Autodesk Inventor part; units mm, degrees
ref_plane "YZ Plane" through (0, 0, 0) normal (1, 0, 0) x (0, 1, 0)
ref_plane "XZ Plane" through (0, 0, 0) normal (0, 1, 0) x (-1, 0, 0)
ref_plane "XY Plane" through (0, 0, 0) normal (0, 0, 1) x (1, 0, 0)
sketch "Sketch1" plane through (0, 0, 0) normal (0, 0, 1) x (1, 0, 0)
  arc A0 (72.4335, -68.9449) -> (-72.4335, -68.9449) centre (0, 0) ccw
  line L0 (0, 0) -> (0, -68.9449)
  arc A1 (75.8476, -68.9449) -> (-75.8476, -68.9449) centre (0, 0) ccw
  line L1 (0, 0) -> (88.7676, -51.25)
  line L2 (0, 0) -> (102.5, 0) construction
  line L3 (0, 0) -> (-88.7676, -51.25)
  line L4 (0, 0) -> (102.5, 0) construction
  line L5 (0, 0) -> (72.4784, 72.4784)
  line L6 (0, 0) -> (102.5, 0) construction
  line L7 (0, 0) -> (-72.4784, 72.4784)
  line L8 (0, 0) -> (102.5, 0) construction
  line L9 (0, 0) -> (-68.416, -39.5)
  line L10 (0, 0) -> (68.416, -39.5)
  line L11 (0, 0) -> (55.8614, 55.8614)
  line L12 (0, 0) -> (-55.8614, 55.8614)
  line L13 (-68.416, -39.5) -> (-51.416, -68.9449)
  line L14 (-68.416, -39.5) -> (-85.416, -10.0551)
  line L15 (68.416, -39.5) -> (51.416, -68.9449)
  line L16 (51.416, -68.9449) -> (68.416, -39.5)
  line L17 (68.416, -39.5) -> (85.416, -10.0551)
  line L18 (-51.416, -68.9449) -> (-75.8476, -68.9449)
  line L19 (-51.416, -68.9449) -> (51.416, -68.9449)
  line L20 (51.416, -68.9449) -> (75.8476, -68.9449)
  line L21 (85.416, -10.0551) -> (100.7418, -18.9035)
  line L22 (-85.416, -10.0551) -> (-100.7418, -18.9035)
  line L23 (-55.8614, 55.8614) -> (-79.9031, 31.8198)
  line L24 (-55.8614, 55.8614) -> (-31.8198, 79.9031)
  line L25 (55.8614, 55.8614) -> (79.9031, 31.8198)
  line L26 (55.8614, 55.8614) -> (31.8198, 79.9031)
  line L27 (-31.8198, 79.9031) -> (-44.3333, 92.4165)
  line L28 (-79.9031, 31.8198) -> (-92.4165, 44.3333)
  line L29 (31.8198, 79.9031) -> (44.3333, 92.4165)
  line L30 (79.9031, 31.8198) -> (92.4165, 44.3333)
  circle A2 centre (0, 0) radius 125
  line L31 (100.7418, -18.9035) -> (121.1717, -30.6987)
  line L32 (-100.7418, -18.9035) -> (-121.1717, -30.6987)
  line L33 (-92.4165, 44.3333) -> (-109.0975, 61.0142)
  line L34 (-44.3333, 92.4165) -> (-61.0142, 109.0975)
  line L35 (44.3333, 92.4165) -> (61.0142, 109.0975)
  line L36 (92.4165, 44.3333) -> (109.0975, 61.0142)
  circle A3 centre (0, 0) radius 120
  line L37 (-75.8476, -68.9449) -> (-104.267, -68.9449)
  line L38 (75.8476, -68.9449) -> (104.267, -68.9449)
  line L39 (68.416, -39.5) -> (86.416, -8.3231)
  line L40 (86.416, -8.3231) -> (121.6665, -28.675)
  line L41 (55.8614, 55.8614) -> (81.3173, 30.4056)
  line L42 (81.3173, 30.4056) -> (111.6152, 56.2764)
  line L43 (-68.416, -39.5) -> (-86.416, -8.3231)
  line L44 (-86.416, -8.3231) -> (-121.6665, -28.675)
  line L45 (-55.8614, 55.8614) -> (-81.3173, 30.4056)
  line L46 (-81.3173, 30.4056) -> (-110.0992, 59.1875)
  line L47 (-55.8614, 55.8614) -> (-30.4056, 81.3173)
  line L48 (-30.4056, 81.3173) -> (-59.1875, 110.0992)
  line L49 (55.8614, 55.8614) -> (30.4056, 81.3173)
  line L50 (30.4056, 81.3173) -> (59.1875, 110.0992)
  line L51 (68.416, -39.5) -> (50.416, -70.6769)
  line L52 (-68.416, -39.5) -> (-50.416, -70.6769)
  line L53 (51.416, -68.9449) -> (87.1717, -89.5884)
  line L54 (51.416, -68.9449) -> (92.7032, -68.9449) construction
  line L55 (50.416, -70.6769) -> (85.6665, -91.0288)
  line L56 (-50.416, -70.6769) -> (-85.6665, -91.0288)
  line L57 (-51.416, -68.9449) -> (-87.1717, -89.5884)
  point P0 (93.8835, 41.1356)
  point P1 (91.8949, 39.4376)
  point P2 (98.796, -15.4707)
  point P3 (101.1125, -16.8081)
  point P4 (40.5138, 91.4255)
  point P5 (42.4052, 93.3169)
  point P6 (-42.4052, 93.3169)
  point P7 (-40.5138, 91.4255)
  point P8 (-91.4255, 40.5138)
  point P9 (-93.3169, 42.4052)
  point P10 (-101.1125, -16.8081)
  point P11 (-98.796, -15.4707)
  point P12 (98.2171, -68.9449)
  point P13 (98.4432, -17.5764)
  point P14 (116.6644, -28.0964)
  point P15 (57.334, 105.4173)
  point P16 (105.4173, 57.334)
  point P17 (-105.4173, 57.334)
  point P18 (-57.334, 105.4173)
  point P19 (-98.2171, -68.9449)
  point P20 (-116.6644, -28.0964)
  point P21 (90.5398, 42.4565)
  point P22 (42.4565, 90.5398)
  point P23 (-42.4565, 90.5398)
  point P24 (-90.5398, 42.4565)
  point P25 (-98.4432, -17.5764)
  point P26 (-86.6025, -50)
  point P27 (-82.6644, -86.9862)
  point P28 (82.6644, -86.9862)
  dimension "d30" = 250
  dimension "d7" = 30
  dimension "d8" = 150
  dimension "d9" = 45
  dimension "d10" = 135
  dimension "d11" = 79
  dimension "d12" = 79
  dimension "d13" = 79
  dimension "d14" = 79
  dimension "d15" = 34
  dimension "d16" = 90
  dimension "d17" = 34
  dimension "d18" = 34
  dimension "d19" = 34
  dimension "d20" = 34
  dimension "d21" = 34
  dimension "d22" = 34
  dimension "d23" = 34
  dimension "d24" = 34
  dimension "d31" = 240
  dimension "d32" = 36
  dimension "d33" = 36
  dimension "d34" = 36
  dimension "d35" = 36
  dimension "d36" = 36
  dimension "d37" = 36
  dimension "d73" = 36
  dimension "d74" = 36
  dimension "d75" = 30
extrude "Extrusion3" add sketch "Sketch1" against normal blind 2 contours L20 L15 L1 A0 | A0 L1 A1 L20 | L1 L17 L21 A0 | A0 L21 A1 L1 | L19 L0 L1 L15 | L21 L39 L40 A0 | A0 L40 A1 L21 | L1 L5 L25 L41 L42 A0 L40 L39 L17 | L19 L13 L3 L0 | A0 L42 A1 L40 | L7 L24 L47 L48 A0 L50 L49 L26 L5 | L3 L14 L43 L44 A0 L46 L45 L23 L7 | L18 A0 L3 L13 | L42 L41 L30 A0 | A0 L30 A1 L42 | L3 A0 L22 L14 | L26 L29 A0 L5 | L5 A0 L30 L25 | L23 L28 A0 L7 | L7 A0 L27 L24 | L18 A1 L3 A0 | A0 L5 A1 L30 | L3 A1 L22 A0 | L22 A0 L44 L43 | A0 L29 A1 L5 | L49 L50 A0 L29 | L7 A1 L27 A0 | A0 L28 A1 L7 | L45 L46 A0 L28 | L27 A0 L48 L47 | L22 A1 L44 A0 | A0 L50 A1 L29 | L27 A1 L48 A0 | A0 L46 A1 L28 | L44 A1 L46 A0 | A0 L48 A1 L50
extrude "Extrusion4" add sketch "Sketch1" along normal blind 28 contours A0 L1 A1 L20 | A0 L21 A1 L1 | A0 L40 A1 L21 | A0 L42 A1 L40 | A0 L30 A1 L42 | L18 A1 L3 A0 | A0 L5 A1 L30 | L3 A1 L22 A0 | A0 L29 A1 L5 | L7 A1 L27 A0 | A0 L28 A1 L7 | L22 A1 L44 A0 | A0 L50 A1 L29 | L27 A1 L48 A0 | A0 L46 A1 L28 | L44 A1 L46 A0 | A0 L48 A1 L50
extrude "Extrusion5" add sketch "Sketch1" along normal blind 65 contours A0 L42 A1 L40 | L44 A1 L46 A0 | A0 L48 A1 L50
sketch "Sketch4" plane through (0, 0, -2) normal (0, 0, -1) x (-1, 0, 0)
  line L0 (0, 0) -> (-85, 0)
  line L1 (0, 0) -> (0, 85)
  line L2 (0, 0) -> (85, 0)
  circle A0 centre (-85, 0) radius 1.5
  circle A1 centre (0, 85) radius 1.5
  circle A2 centre (85, 0) radius 1.5
  circle A3 centre (0, 0) radius 75
  dimension "d60" = 85
  dimension "d61" = 85
  dimension "d62" = 85
  dimension "d63" = 3
  dimension "d64" = 3
  dimension "d65" = 3
  dimension "d66" = 150
extrude "Extrusion11" cut sketch "Sketch4" against normal blind 45
sketch "Sketch5" plane through (0, 0, -2) normal (0, 0, -1) x (-1, 0, 0)
  line L0 (72.4335, -68.9449) -> (-72.4335, -68.9449)
  line L1 (-72.4335, -68.9449) -> (-72.4335, -54.9449)
  line L2 (-72.4335, -54.9449) -> (129.3344, -54.9449)
  line L3 (129.3344, -54.9449) -> (-118.857, -54.9449)
  line L4 (-118.857, -54.9449) -> (-118.857, -84.9238)
  line L5 (-118.857, -84.9238) -> (129.3344, -84.9238)
  line L6 (129.3344, -84.9238) -> (129.3344, -54.9449)
  point P0 (0, 0)
  point P1 (-41.6566, -68.9449)
  dimension "d70" = 14
extrude "Extrusion12" cut sketch "Sketch5" against normal blind 4
properties part number "Falda-Parte1"
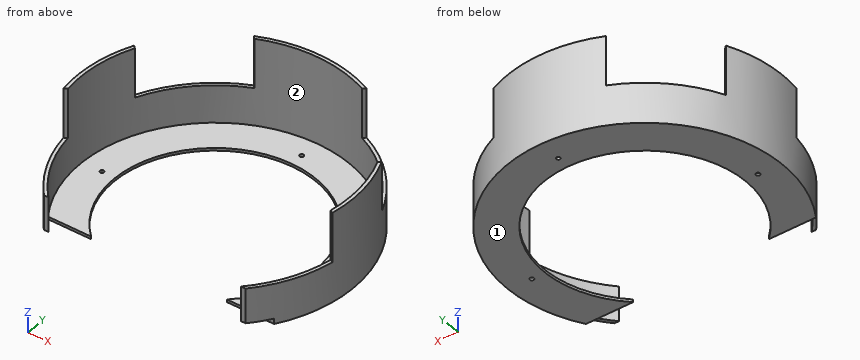
Read the model definition and answer for the solid it produces. Units are mm, in the model's axes. Face numbers are marked on the shaded views. A direction names the side the tool comes from. Give positions to 0.01 mm unless a question says otherwise; leave off trailing zeros. Order: outer loops, then holes, each group sorted by start corner. A loop starts at its lowest first (then second) coordinate and runs counter-clockwise, first axis right, second up.
(1) Find section D-D (x = -8). Give the vertices of the cut face in (y, z).
(2) Straight lines are drawn through the part: L1, parallel to Y at x = 0, z = -0.9; L2, parallel to X at y = 0, z = 17; L3, parallel to X at y = -8.5, z = 26. For each, find the intervals that lie inside material, in ascending order.
(3) Find section B-B (z = 36). Give the vertices of the cut face in (x, y), plus the area to 3 significant figures.
(4) Find section A-A (y = -45). Give the vertices of the cut face in (x, z).
(5) Find section C-C (y = -5). Give the vertices of the cut face in (x, z).
(6) Given pin 1 (4 mm diameter, centred on x = -81.5, y = -64, fed in from -Z); pin 2 (3 mm diameter, centred on x = 23, z = 45, fed in from +Y); pin 3 (14.5 mm diameter, centred on x = -83, y = -40, fed in from +Z); pin 4 (3.5 mm diameter, centred on x = 0, y = 85, fed in from -Z), each flat-ended and moving along its own axis, determine where each tip first touches the part or whether it passes through.
(7) For the marked faces 1 and 2, determine the directions among +Z, -Z, +X, -X, +Y, -Y from which every point of the face is accessible in a straight line to the end or side of a thin tool.
Result sheet:
1. outline: (74.57, -2) - (102.19, -2) - (102.19, 65) - (99.68, 65) - (99.68, 0) - (74.57, 0) - close
2. L1: y = 75 to 83.5, 86.5 to 102.5
2. L2: x = -102.5 to -100, 100 to 102.5
2. L3: x = -102.15 to -99.64, 99.64 to 102.15
3. outline: (-101.11, -16.81) - (-98.8, -15.47) arc R100 cw to (-91.43, 40.51) - (-93.32, 42.41) arc R102.5 ccw to start; (-42.41, 93.32) - (-40.51, 91.43) arc R100 cw to (40.51, 91.43) - (42.41, 93.32) arc R102.5 ccw to start; (91.89, 39.44) arc R100 cw to (98.8, -15.47) - (101.11, -16.81) arc R102.5 ccw to (93.88, 41.14) - close
3. area: 505 mm2
4. outline: (-92.09, -2) - (-60, -2) - (-60, 0) - (-89.3, 0) - (-89.3, 28) - (-92.09, 28) - close; (60, -2) - (92.09, -2) - (92.09, 28) - (89.3, 28) - (89.3, 0) - (60, 0) - close
5. outline: (-102.38, -2) - (-74.83, -2) - (-74.83, 0) - (-99.87, 0) - (-99.87, 65) - (-102.38, 65) - close; (74.83, -2) - (102.38, -2) - (102.38, 65) - (99.87, 65) - (99.87, 0) - (74.83, 0) - close
6. pin 1: stops at z = 2
6. pin 2: stops at y = 100.22
6. pin 3: stops at z = 0
6. pin 4: stops at z = -2
7. face 1: -Z, +X, -X, +Y, -Y
7. face 2: +Z
